The drawing under review shows one solid part. Ordinate dimensions are in mm from its lowest x, y, z. A direction names the side the tool comes from. Round coordinates to 2 decimals unless told otherwise and drop trailing zeros. Order: outer loops, then holes, each group sorted by start corner. A loop starts at its lowest first (then second) coordinate and runs counter-clockwise, first axis right, second up.
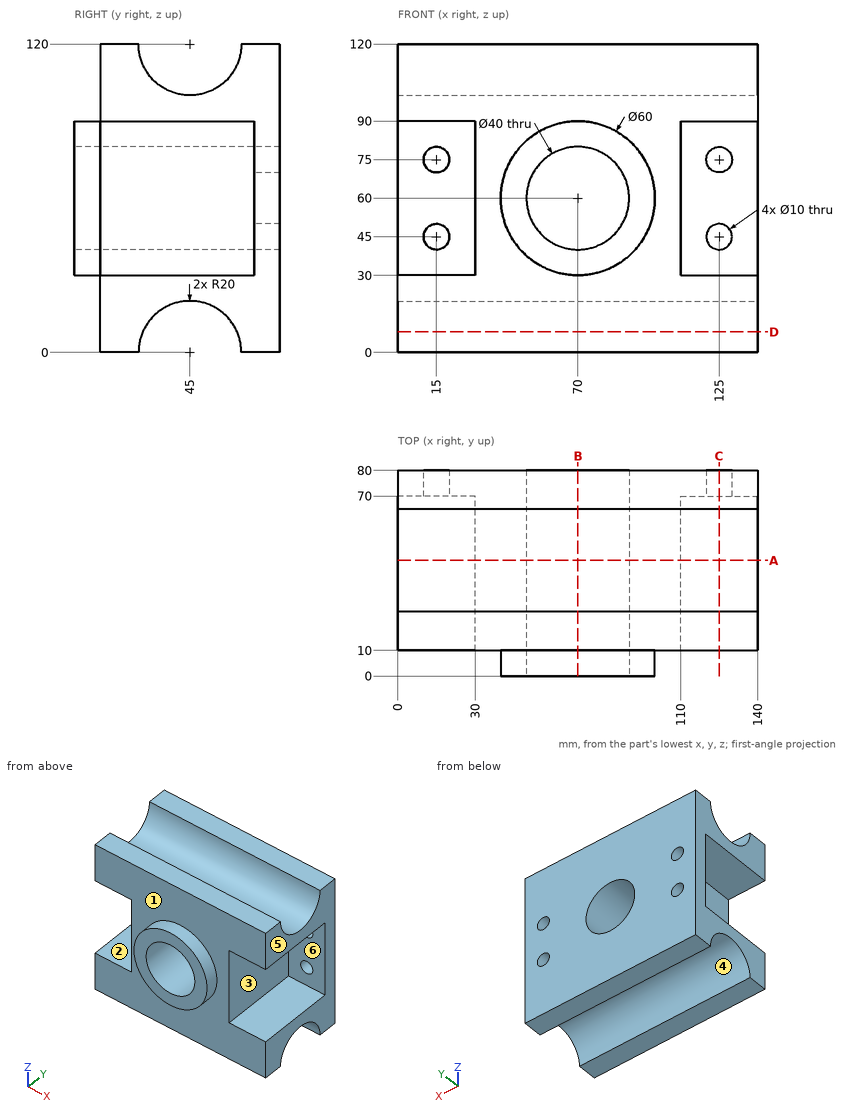
(1) We need section B-B (x = 70). Give the boundary of the cut face in (y, z).
(2) Tool access review of the marked faces 1, 2 and 3: name each direction out of +Z, -Z, +X, -X, +Y, -Y from which nothing blocks a thin tool from reaching the whole face with its end or side.
(3) We need section C-C (x = 125). Give the boundary of the cut face in (y, z).
(4) Clearance check with flat-ended pins moving along their axes: P1, Ø3, axis at x = 22.5, z = 50.5, coming from the -Y side; P2, Ø12, axis at x = 75, y = 37, coming from the -Z side; P3, Ø6, axis at x = 107, y = 43.5, coming from the +Z side. State where each tip first meets the part, or that it passes through.
(5) We need section D-D (z = 8). Give the boundary of the cut face in (x, y), and give its area (3 significant figures).
(6) The part is to be moulded in two halves that separate along Y. For the marked faces 4, 5 and 6, say which applies: pulls with the +Y half, pulls with the -Y half, needs draft (parallel to the pull), parting line crosses it, or undercut.
(7) To check wall thickness, follow L1, parallel to Z at x = 15, y = 77.25; L2, parallel to X at y = 72, z = 75; L3, parallel to Y at x = 123.5, z = 21. State the ranges of each line that lie inside material, in increasing order.
(8) We need section A-A (y = 45). Give the boundary of the cut face in (x, z), and give its area (3 significant figures).
Verdict:
1. outline: (0, 30) - (10, 30) - (10, 0) - (25, 0) arc R20 cw to (65, 0) - (80, 0) - (80, 40) - (0, 40) - close; (0, 80) - (80, 80) - (80, 120) - (65, 120) arc R20 cw to (25, 120) - (10, 120) - (10, 90) - (0, 90) - close
2. face 1: -Y
2. face 2: -X, -Y
2. face 3: +X, -Y
3. outline: (10, 0) - (25, 0) arc R20 cw to (65, 0) - (80, 0) - (80, 40) - (70, 40) - (70, 30) - (10, 30) - close; (10, 90) - (70, 90) - (70, 80) - (80, 80) - (80, 120) - (65, 120) arc R20 cw to (25, 120) - (10, 120) - close; (70, 50) - (80, 50) - (80, 70) - (70, 70) - close
4. P1: stops at y = 70
4. P2: stops at z = 14.28
4. P3: stops at z = 100.51
5. outline: (0, 10) - (140, 10) - (140, 26.67) - (0, 26.67) - close; (0, 63.33) - (140, 63.33) - (140, 80) - (0, 80) - close
5. area: 4,670 mm2
6. face 4: undercut
6. face 5: needs draft
6. face 6: pulls with the -Y half
7. L1: z = 0 to 40, 50 to 70, 80 to 120
7. L2: x = 0 to 10, 20 to 56.77, 83.23 to 120, 130 to 140
7. L3: y = 10 to 80
8. outline: (0, 20) - (140, 20) - (140, 30) - (110, 30) - (110, 90) - (140, 90) - (140, 100) - (0, 100) - (0, 90) - (30, 90) - (30, 30) - (0, 30) - close; hole circle Ø40 at (70, 60)
8. area: 6,340 mm2
